```python
from build123d import *

# Parameters (mm, degrees)
PAD_DEPTH      = 380
PAD_DEPTH_BACK = 380
FILLET_R       = 10


with BuildPart() as part:
    # Sketch → Pad (new body, two sides)
    with BuildSketch(Plane.YZ) as pad_sk:
        Polygon((-380, 0), (-480, 100), (0, 100), (0, 0), align=None)
    extrude(amount=PAD_DEPTH)
    extrude(pad_sk.sketch, amount=-PAD_DEPTH_BACK)

    # Fillet
    fillet_edges = [part.edges().sort_by_distance(p)[0] for p in [
        (0, -480, 100),
        (0, 0, 100),
        (-380, -240, 100),
        (380, -240, 100),
        (0, -380, 0),
        (-380, -430, 50),
        (380, -430, 50),
        (380, 0, 50),
        (380, -190, 0),
        (0, 0, 0),
        (-380, 0, 50),
        (-380, -190, 0),
    ]]
    fillet(fillet_edges, radius=FILLET_R)


solid = part.part
```
Can you work these out from the model? Positions are in its coordinate system, mm. Give positions to 0.01 mm unless a question says otherwise; leave off trailing zeros. Loops run counter-clockwise (first coordinate to the right, second up) from the corner with the lowest first, then second, coordinate; pieces in that order, holes last. Notation, with made-up numbers: M -26.75,0 L 23.25,0 A17 ccw 23.25,7 Z; hole C 86.5,59.25 d7. An arc over 180 degrees is marked long. One line per item, written item: value.
(1) I need wall thicknesses on line 1 (Y direction, x = 86, z = 76); line 2 (Y direction, x = 315.5, z = 61); line 3 (Z direction, x = 104, y = -434). Which ranges of each line are inside material? Lowest first, please.
Returned:
line 1: -456 to 0
line 2: -441 to 0
line 3: 54 to 100
(2) Will these pins go through, and if not, where does the flat tip stop? pin 1 (8 mm diameter, centred on x = 147.5, z = 74, fed in from -Y); pin 2 (2 mm diameter, centred on x = -14, z = 18, fed in from -Y); pin 3 (1.5 mm diameter, centred on x = 212, y = -167, fed in from -Z); pin 4 (6 mm diameter, centred on x = -226.5, z = 35, fed in from -Y).
Returned:
pin 1: y = -458
pin 2: y = -399
pin 3: z = 0
pin 4: y = -418
(3) Suppose I cut it at A-A on x = 260.5. List the corners of the cut face in (y, z) for me, plus the area to 3 significant figures.
Returned:
outline: M -462.93,82.93 L -382.93,2.93 A10 ccw -375.86,0 L -10,0 A10 ccw 0,10 L 0,90 A10 ccw -10,100 L -455.86,100 A10 ccw Z
area: 42,800 mm^2
